Source: CAD feature listing. Evaluate the final solid. Frame: model axes, mm. A direction names the side the tool comes from. Round coordinates to 2 decimals unless told otherwise and drop trailing zeros. Write each loop counter-clockwise with the first axis right and the second up, starting at its lowest first coordinate (ties: lowest second). Pieces come first, ordered by that corner, then holes. Notation, with made-up numbers: (84, -23) -> (103, -23) arc R13 cw to (103, 2) -> close; hole circle Ø1 at (-22, 58). An arc over 180 degrees is marked (long way). Return JSON: item names as keys, results as strings. Group by question number.
from build123d import *

# Parameters (mm, degrees)
PAD_DEPTH       = 58
SKETCH001_R     = 9.5
SKETCH001_R_2   = 7.6
PAD001_DEPTH    = 58
SKETCH002_R     = 7.6
SKETCH002_R_2   = 3
POCKET_DEPTH    = 58
SKETCH003_R     = 4.1
SKETCH003_W     = 9
SKETCH003_H     = 33
POCKET001_DEPTH = 55
SKETCH004_W     = 16
SKETCH004_H     = 13
POCKET002_DEPTH = 45
PAD002_DEPTH    = 58
SKETCH006_R     = 1.6
POCKET003_DEPTH = 17
SKETCH007_W     = 18
SKETCH007_H     = 58
POCKET004_DEPTH = 25
SKETCH008_W     = 17
SKETCH008_H     = 33
POCKET005_DEPTH = 5
SKETCH009_W     = 7
SKETCH009_H     = 33
POCKET006_DEPTH = 5
SKETCH010_W     = 8
SKETCH010_H     = 49
POCKET007_DEPTH = 45
SKETCH011_W     = 4
SKETCH011_H     = 17
POCKET008_DEPTH = 20
POCKET009_DEPTH = 58
SKETCH013_W     = 20
SKETCH013_H     = 5.8
SKETCH013_W_2   = 17.2
SKETCH013_H_2   = 1.8
PAD003_DEPTH    = 6
SKETCH014_W     = 17
SKETCH014_H     = 6
POCKET010_DEPTH = 3.8
SKETCH015_R     = 1.7
POCKET011_DEPTH = 27.001
FILLET_R        = 1
FILLET001_R     = 4


with BuildPart() as part:
    # Sketch → Pad (new body)
    with BuildSketch(Plane(origin=(-133, 0, 90), x_dir=(1, 0, 0), z_dir=(0, 0, 1))):
        Polygon((-47.676132, 21.976631), (5.323868, 21.976631), (5.323868, 5.976631), (-12.676132, 5.976631), (-12.676132, -0.023369), (-16.676132, -7.023369), (-24.676132, -7.023369), (-31.676132, 5.976631), (-47.676132, 5.976631), align=None)
    extrude(amount=PAD_DEPTH)

    # Sketch001 → Pad001 (new body)
    with BuildSketch(Plane(origin=(-133, 0, 148), x_dir=(1, 0, 0), z_dir=(0, 0, 1))):
        with Locations((-38.176132, -0.523369)):
            Circle(SKETCH001_R)
        with Locations((-38.176132, -0.523369)):
            Circle(SKETCH001_R_2, mode=Mode.SUBTRACT)
    extrude(amount=-PAD001_DEPTH)

    # Sketch002 → Pocket (cut)
    with BuildSketch(Plane(origin=(-133, 0, 148), x_dir=(1, 0, 0), z_dir=(0, 0, 1))):
        with Locations((-38.176132, -0.523369)):
            Circle(SKETCH002_R)
        with Locations((-21.176132, -0.523369)):
            Circle(SKETCH002_R_2)
    extrude(amount=-POCKET_DEPTH, mode=Mode.SUBTRACT)

    # Sketch003 → Pocket001 (cut)
    with BuildSketch(Plane(origin=(-180.676132, 0, 90), x_dir=(0, -1, 0), z_dir=(-1, 0, 0))):
        with Locations((-13.476631, 52)):
            Circle(SKETCH003_R)
        with Locations((-13.476631, 7)):
            Circle(SKETCH003_R)
        with Locations((-13.676631, 29.5)):
            Rectangle(SKETCH003_W, SKETCH003_H)
    extrude(amount=-POCKET001_DEPTH, mode=Mode.SUBTRACT)

    # Sketch004 → Pocket002 (cut)
    with BuildSketch(Plane(origin=(-133, 0, 148), x_dir=(1, 0, 0), z_dir=(0, 0, 1))):
        with Locations((-20.676132, -0.523369)):
            Rectangle(SKETCH004_W, SKETCH004_H)
    extrude(amount=-POCKET002_DEPTH, mode=Mode.SUBTRACT)

    # Sketch005 → Pad002 (new body)
    with BuildSketch(Plane(origin=(-133, 0, 148), x_dir=(1, 0, 0), z_dir=(0, 0, 1))):
        Polygon((-47.676132, 21.976631), (-91.676132, 21.976631), (-91.676132, 11.976631), (-81.676132, 11.976631), (-47.676132, 5.976631), align=None)
    extrude(amount=-PAD002_DEPTH)

    # Sketch006 → Pocket003 (cut)
    with BuildSketch(Plane(origin=(-133, 21.976631, 90), x_dir=(-1, 0, 0), z_dir=(0, 1, 0))):
        with Locations((56.676132, 44.5)):
            Circle(SKETCH006_R)
        with Locations((56.676132, 13.5)):
            Circle(SKETCH006_R)
        with Locations((87.676132, 13.5)):
            Circle(SKETCH006_R)
        Polygon((91.676132, 18), (81.676132, 18), (81.676132, 16), (59.676132, 16), (59.676132, 39), (61.676132, 39), (61.676132, 49), (47.676132, 49), (47.676132, 58), (91.676132, 58), align=None)
    extrude(amount=-POCKET003_DEPTH, mode=Mode.SUBTRACT)

    # Sketch007 → Pocket004 (cut)
    with BuildSketch(Plane(origin=(-133, 5.976631, 90), x_dir=(1, 0, 0), z_dir=(0, -1, 0))):
        with Locations((-3.676132, 29)):
            Rectangle(SKETCH007_W, SKETCH007_H)
    extrude(amount=-POCKET004_DEPTH, mode=Mode.SUBTRACT)

    # Sketch008 → Pocket005 (cut)
    with BuildSketch(Plane(origin=(-133, 21.976631, 90), x_dir=(-1, 0, 0), z_dir=(0, 1, 0))):
        with Locations((30.176132, 29.5)):
            Rectangle(SKETCH008_W, SKETCH008_H)
    extrude(amount=-POCKET005_DEPTH, mode=Mode.SUBTRACT)

    # Sketch009 → Pocket006 (cut)
    with BuildSketch(Plane(origin=(-133, 5.976631, 90), x_dir=(1, 0, 0), z_dir=(0, -1, 0))):
        with Locations((-25.176132, 29.5)):
            Rectangle(SKETCH009_W, SKETCH009_H)
    extrude(amount=-POCKET006_DEPTH, mode=Mode.SUBTRACT)

    # Sketch010 → Pocket007 (cut)
    with BuildSketch(Plane(origin=(-224.676132, 0, 90), x_dir=(0, -1, 0), z_dir=(-1, 0, 0))):
        with Locations((-9.976631, 24.5)):
            Rectangle(SKETCH010_W, SKETCH010_H)
    extrude(amount=-POCKET007_DEPTH, mode=Mode.SUBTRACT)

    # Sketch011 → Pocket008 (cut)
    with BuildSketch(Plane(origin=(-192.676132, 0, 90), x_dir=(0, -1, 0), z_dir=(-1, 0, 0))):
        with Locations((-15.976631, 27.5)):
            Rectangle(SKETCH011_W, SKETCH011_H)
    extrude(amount=-POCKET008_DEPTH, mode=Mode.SUBTRACT)

    # Sketch012 → Pocket009 (cut)
    with BuildSketch(Plane(origin=(-133, 0, 148), x_dir=(1, 0, 0), z_dir=(0, 0, 1))):
        Polygon((-38.722618, -1.360837), (-49.563332, 5.713227), (-49.016846, 6.550695), (-38.176132, -0.523369), align=None)
    extrude(amount=-POCKET009_DEPTH, mode=Mode.SUBTRACT)

    # Sketch013 → Pad003 (new body)
    with BuildSketch(Plane(origin=(-133, 0, 148), x_dir=(1, 0, 0), z_dir=(0, 0, 1))):
        with Locations((-22.676132, 14.076631)):
            Rectangle(SKETCH013_W, SKETCH013_H)
        with Locations((-22.076132, 14.076631)):
            Rectangle(SKETCH013_W_2, SKETCH013_H_2, mode=Mode.SUBTRACT)
    extrude(amount=PAD003_DEPTH)

    # Sketch014 → Pocket010 (cut)
    with BuildSketch(Plane(origin=(-133, 11.176631, 90), x_dir=(1, 0, 0), z_dir=(0, -1, 0))):
        with Locations((-21.176132, 61)):
            Rectangle(SKETCH014_W, SKETCH014_H)
    extrude(amount=-POCKET010_DEPTH, mode=Mode.SUBTRACT)

    # Sketch015 → Pocket011 (cut, through all)
    with BuildSketch(Plane(origin=(-133, 16.976631, 90), x_dir=(-1, 0, 0), z_dir=(0, 1, 0))):
        with Locations((15.676132, 61)):
            Circle(SKETCH015_R)
    extrude(amount=-POCKET011_DEPTH, mode=Mode.SUBTRACT)

    # Fillet
    fillet_edges = [part.edges().sort_by_distance(p)[0] for p in [
        (-224.676132, 17.976631, 108),
        (-194.676132, 17.976631, 129),
        (-214.676132, 17.976631, 108),
    ]]
    fillet(fillet_edges, radius=FILLET_R)

    # Fillet001
    fillet001_edges = [part.edges().sort_by_distance(p)[0] for p in [
        (-194.676132, 17.976631, 139),
    ]]
    fillet(fillet001_edges, radius=FILLET001_R)


solid = part.part
Item 1: Cut plane D-D on z = 122. Output: boundary loops of the cut face in (x, y), and give its area (3 significant figures).
Item 2: Material intervals for probe 1 along X at (y, z) = (16.5, 103.5); probe 2 along X at (y, z) = (19.5, 134.5); probe 3 along X at (y, z) = (8, 119), sorted ascending.
Item 3: Cut plane C-C on z = 144. Output: boundary loops of the cut face in (x, y), and give its area (3 significant figures).
Item 4: Set-up query: faces 1 (the flat face through (-165.676, 14, 151)), 2 (the flat face through (-180.676, 16, 127)), 3 (the flat face through (-187, 16, 109)), 4 (the flat face through (-178.82, 3.27, 119.41)). Return all of +Z, -Z, +X, -X, +Y, -Y with unobstructed straight access to the full face (end or side cutting, diameter ignored); none if empty.
Item 5: Cut plane B-B on x = -153.5. Output: boundary loops of the cut face in (y, z).
Item 6: First-contact query: pin 1 Ø10 at (x, z) = (-202.5, 100) entering from -Y; pin 2 Ø9 at (y, z) = (10, 112.5) entering from -X; pin 3 Ø2 at (y, z) = (14.5, 152) entering from +X; pin 4 Ø5 at (x, z) = (-158, 152) entering from +Y. Flat tips, straight axial feed; report the tip coordinate or a pass-through.
Item 7: Pull-direction query (Y, two-part tool) for faces 5 (the flat face through (-179, 5.977, 119)), 6 (the flat face through (-154.676, 8, 119)), 7 (the flat face through (-147.648, -3.474, 96.409)); classes: +Y half, -Y half, draft (parallel to the pull), parting line (faces both ways), or undercut.
Item 8: Cut plane A-A on y = 19.5. Output: boundary loops of the cut face in (x, z), and give its area (3 significant figures).
Here are the results:
{
 "1": {"outline": "(-192.68, 17.98) -> (-180.68, 17.98) -> (-180.68, 18.18) -> (-171.68, 18.18) -> (-171.68, 21.98) -> (-192.68, 21.98) -> close; (-179.68, 5.98) -> (-178.1, 5.98) arc R9.5 ccw to (-179.13, 4.67) -> (-177.54, 3.63) arc R7.6 cw (long way) to (-178.03, 2.76) -> (-179.63, 3.8) arc R9.5 ccw (long way) to (-161.73, 0.51) -> (-161.68, 0.41) -> (-161.68, 9.18) -> (-179.68, 9.18) -> close; (-154.68, 5.98) -> (-145.68, 5.98) -> (-145.68, 9.18) -> (-154.68, 9.18) -> close; (-154.68, 18.18) -> (-145.68, 18.18) -> (-145.68, 21.98) -> (-154.68, 21.98) -> close", "area": "279 mm^2"},
 "2": {"probe 1": "x = -224.68 to -222.28, -219.08 to -191.28, -188.08 to -180.68", "probe 2": "x = -194.68 to -191.28, -188.08 to -171.68, -154.68 to -145.68", "probe 3": "x = -179.68 to -161.68, -154.68 to -145.68"},
 "3": {"outline": "(-180.68, 5.98) -> (-178.1, 5.98) arc R9.5 ccw to (-179.13, 4.67) -> (-177.54, 3.63) arc R7.6 cw (long way) to (-178.03, 2.76) -> (-179.63, 3.8) arc R9.5 ccw (long way) to (-161.73, 0.51) -> (-161.68, 0.41) -> (-161.68, 5.98) -> (-145.68, 5.98) -> (-145.68, 9.9) -> (-180.68, 9.9) -> close; (-180.68, 17.06) -> (-145.68, 17.06) -> (-145.68, 21.98) -> (-180.68, 21.98) -> close", "area": "386 mm^2"},
 "4": {"face 1": "+Z, -X, +Y, -Y", "face 2": "+X", "face 3": "+X, -X, -Y", "face 4": "+Z, -Z"},
 "5": {"outline": "(-7.02, 90) -> (-3.45, 90) -> (-3.45, 103) -> (-7.02, 103) -> close; (2.4, 90) -> (21.98, 90) -> (21.98, 148) -> (16.98, 148) -> (16.98, 154) -> (14.98, 154) -> (14.98, 148) -> (5.98, 148) -> (5.98, 103) -> (2.4, 103) -> close; hole (9.18, 103) -> (18.18, 103) -> (18.18, 136) -> (9.18, 136) -> close; hole circle Ø8.2 at (13.48, 97); hole circle Ø8.2 at (13.48, 142)"},
 "6": {"pin 1": "stops at y = 13.98", "pin 2": "stops at x = -179.68", "pin 3": "stops at x = -145.68", "pin 4": "stops at y = 16.98"},
 "7": {"face 5": "undercut", "face 6": "draft", "face 7": "-Y half"},
 "8": {"outline": "(-224.68, 90) -> (-145.68, 90) -> (-145.68, 148) -> (-180.68, 148) -> (-180.68, 139) -> (-190.68, 139) arc R4 ccw to (-194.68, 135) -> (-194.68, 130) arc R1 ccw to (-193.68, 129) -> (-192.68, 129) -> (-192.68, 106) -> (-214.68, 106) -> (-214.68, 107) arc R1 ccw to (-215.68, 108) -> (-223.68, 108) arc R1 ccw to (-224.68, 107) -> close; hole circle Ø3.2 at (-220.68, 103.5); hole circle Ø3.2 at (-189.68, 103.5); hole circle Ø3.2 at (-189.68, 134.5); hole (-171.68, 103) -> (-154.68, 103) -> (-154.68, 136) -> (-171.68, 136) -> close", "area": "2,580 mm^2"}
}
